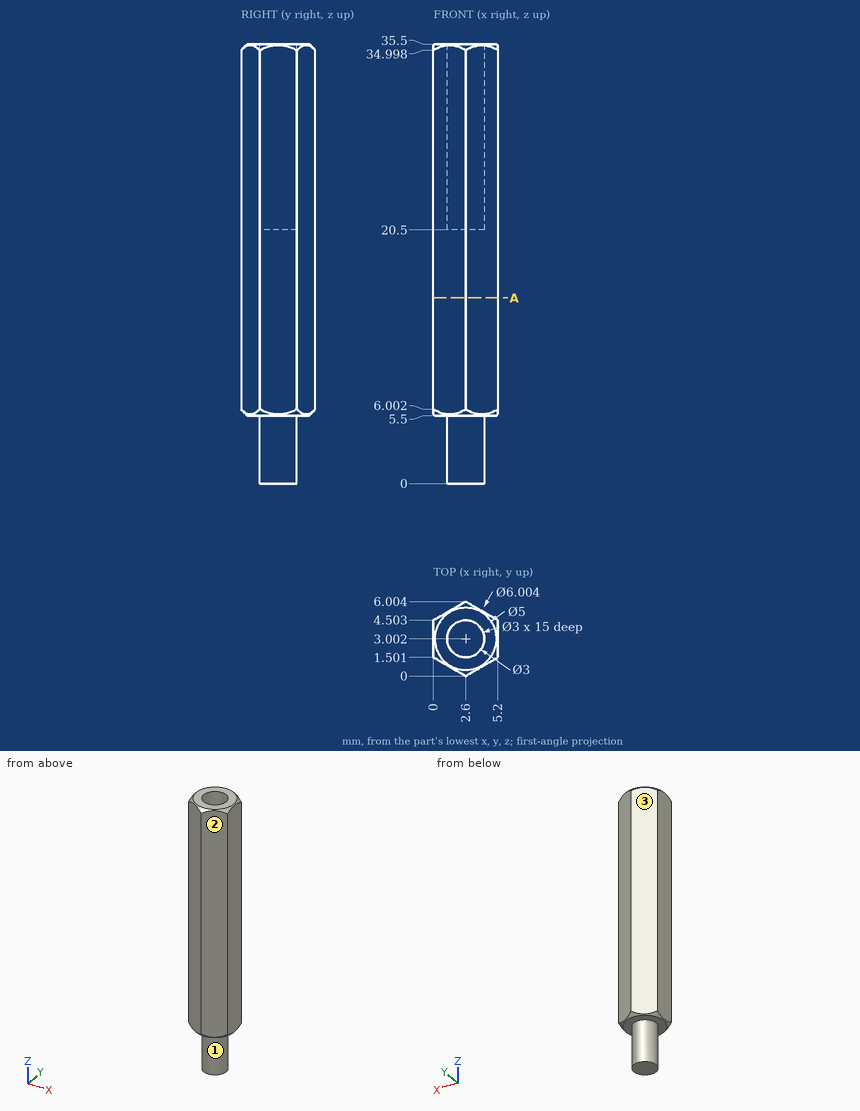
Check sheet for the drawn part. Datum: minimum x, y, z corner. Units: mm. Round coordinates to 2 decimals unless told otherwise and drop trailing zeros. Loops run counter-clockwise (first coordinate to the right, second up) from the corner with the lowest first, then second, coordinate; pieces in that order, holes last. Notation, with made-up numbers: M 53,13.25 L 80,13.25 A13 ccw 80,37.25 Z; hole C 3,-29 d8. An arc over 180 degrees is marked long. One line per question, with ' | ' between items. Start each with the question number.
Item 1: Gauge pin test, flat end, axial feed: pin 1 Ø1.5 at (x, y) = (2.5, 3) entering from +Z. Record the tip position at first contact, or that the pin passes through.
Item 2: Scan lines: probe 1 along X at (y, z) = (2, 32) (1 decimal); probe 2 along Z at (x, y) = (4.8, 3); probe 3 along Z at (x, y) = (2.7, 3.5). Record each from-to range of solid material in increasing order.
Item 3: Release check for a two-part mould opening along X. For the marked faces 1, 2 and 3 record: released by +X, released by -X, zero draft, split by the parting line, or undercut.
Item 4: Section check A-A (z = 15). Record the boundary of the cut face in (x, y) (1 decimal), and give its area (3 significant figures).
Worked out:
1) pin 1: z = 20.5
2) probe 1: 0 to 1.5, 3.7 to 5.2 | probe 2: 5.5 to 35.5 | probe 3: 0 to 20.5
3) face 1: split by the parting line | face 2: released by +X | face 3: released by -X
4) outline: M 0,1.5 L 2.6,0 L 5.2,1.5 L 5.2,4.5 L 2.6,6 L 0,4.5 Z | area: 23.4 mm^2
